Work out the finished part from the listing and answer in its coordinate system (mm). A direction names the side the tool comes from. Coordinates: 2 decimals unless noted, no trailing zeros. Order: outer loops, then holes, each group sorted by start corner. A loop starts at its lowest first (then second) coordinate and runs counter-clockwise, first axis right, second up. Notation, with made-up numbers: M -21,47 L -10,47 A26 cw -10,81 Z; hole C -0.75,48.25 d8. An arc over 180 degrees is marked long. Use a Markdown table: item, result.
Autodesk Inventor part; units mm, degrees
ref_plane "YZ Plane" through (0, 0, 0) normal (1, 0, 0) x (0, 1, 0)
ref_plane "XZ Plane" through (0, 0, 0) normal (0, 1, 0) x (-1, 0, 0)
ref_plane "XY Plane" through (0, 0, 0) normal (0, 0, 1) x (1, 0, 0)
sketch "スケッチ1" plane through (0, 0, 0) normal (0, 0, 1) x (1, 0, 0)
  line L0 (0, 0) -> (-28.77, 0)
  line L1 (-28.77, 0) -> (-28.77, -33.8125)
  line L2 (-28.77, -33.8125) -> (0, -33.8125)
  line L3 (0, -33.8125) -> (0, 0)
  circle A0 centre (-14.385, -28.04) radius 15.5
  line L4 (0, -4) -> (-5, 0)
  line L5 (-23.77, 0) -> (-28.77, -4)
  dimension "d0" = 28.77
  dimension "d2" = 31
  dimension "d4" = 4
  dimension "d5" = 4
  dimension "d6" = 5
  dimension "d7" = 5
  dimension "d66" = 28.04
extrude "押し出し1" add sketch "スケッチ1" along normal blind 9 contours L4 L3 A0 L1 L5 L0 | L3 L2 L1 A0 | A0 L2
sketch "スケッチ2" plane through (0, 0, 9) normal (0, 0, 1) x (1, 0, 0)
  line L0 (-5, 0) -> (-23.77, 0)
  arc A0 (-28.77, -33.8125) -> (0, -33.8125) centre (-14.385, -28.04) ccw
  point P0 (0, 0)
hole "穴1" at (-14.385, -28.04, 9) direction (0, 0, -1) diameter 8 end through all
sketch "スケッチ3" plane through (0, 0, 9) normal (0, 0, 1) x (1, 0, 0)
  line L0 (-28.77, -33.8125) -> (-38.2682, -31.1712)
  line L1 (-28.77, -22.086) -> (-38.3232, -24.9246)
  circle A0 centre (-37.3975, -28.04) radius 3.25
  circle A1 centre (-14.385, -28.04) radius 4
  line L2 (0, -33.8125) -> (9.4982, -31.1712)
  line L3 (0, -22.086) -> (9.5532, -24.9246)
  circle A2 centre (8.6275, -28.04) radius 3.25
  line L4 (-28.77, -4) -> (-28.77, -33.8125)
  line L5 (0, -33.8125) -> (0, -4)
  point P0 (0, 0)
  dimension "d19" = 5.954
  dimension "d20" = 6.5
  dimension "d53" = 46.025
  dimension "d54" = 23.0125
  dimension "d55" = 6.5
extrude "押し出し2" add sketch "スケッチ3" against normal blind 2.5 contours L0 A0 L1 L4 | A0 | L5 L3 A2 L2 | A2
sketch "スケッチ4" plane through (0, 0, 6.5) normal (0, 0, -1) x (-1, 0, 0)
  arc A0 (0, -33.8125) -> (28.77, -33.8125) centre (14.385, -28.04) ccw
  point P0 (0, 0)
  point P1 (30.6, -28.04)
  point P2 (-1.83, -28.04)
  dimension "d26" = 16.215
  dimension "d27" = 16.215
hole "穴2" at (-30.6, -28.04, 6.5) at (1.83, -28.04, 6.5) direction (0, 0, 1) diameter 3 end through all
sketch "スケッチ5" plane through (0, 0, 6.5) normal (0, 0, -1) x (-1, 0, 0)
  circle A0 centre (30.6, -28.04) radius 1.5
  circle A1 centre (-1.83, -28.04) radius 1.5
  point P0 (0, 0)
hole "穴3" at (-30.6, -28.04, 6.5) at (1.83, -28.04, 6.5) direction (0, 0, 1) diameter 5.6 depth 1.8
sketch "スケッチ6" plane through (0, 0, 6.5) normal (0, 0, -1) x (-1, 0, 0)
  circle A0 centre (14.385, -28.04) radius 4
  point P0 (0, 0)
  point P1 (37.3975, -28.04)
  point P2 (-8.6275, -28.04)
  dimension "d43" = 23.0125
  dimension "d45" = 23.0125
hole "穴4" at (-37.3975, -28.04, 6.5) at (8.6275, -28.04, 6.5) at (-14.385, -28.04, 6.5) direction (0, 0, 1) diameter 2.87 end through all
fillet "フィレット1" radius 0.4 4 edges at (-28.77, -4, 4.5) (-23.77, 0, 4.5) (-5, 0, 4.5) (0, -4, 4.5)
fillet "フィレット2" radius 0.5 10 edges at (-28.7305, -4.019, 0) (-26.2497, -1.9838, 0) (-23.7621, -0.0225, 0) (-14.385, 0, 0) (-5.0079, -0.0225, 0) (-2.5203, -1.9838, 0) (-0.0395, -4.019, 0) (0, -19.0024, 0) (-28.77, -19.0024, 0) (-14.385, -43.54, 0)
sketch "スケッチ7" plane through (-23.6297, 0, 9) normal (0, 1, 0) x (1, 0, 0)
  line L0 (3.2447, 5) -> (15.2447, 5)
  line L1 (15.2447, 5) -> (15.2447, 2)
  line L2 (15.2447, 2) -> (3.2447, 2)
  line L3 (3.2447, 2) -> (3.2447, 5)
  line L4 (18.4894, 0) -> (0, 0)
  point P0 (23.6297, 9)
  dimension "d60" = 3
  dimension "d61" = 12
  dimension "d62" = 8.385
  dimension "d63" = 2
extrude "押し出し3" add sketch "スケッチ7" along normal blind 5
equation "\"d4\" = d5"
equation "\"d6\" = d7"
equation "\"d54\" = 0.5 * d53"
equation "\"d55\" = d20"
properties part number "AMT102-V"
1. Find the intervals of material crossed by probe 1 along X at (y, z) = (-28.04, 8.6) (1 decimal); probe 2 along X at (y, z) = (-28.04, 7.05) (1 decimal); probe 3 along Y at (x, z) = (-30.6, 7.9), in increasing order.
Answers below:
| item | result |
|---|---|
| probe 1 | -40.6 to -38.8, -36 to -32.1, -29.1 to -18.4, -10.4 to 0.3, 3.3 to 7.2, 10.1 to 11.9 |
| probe 2 | -40.6 to -38.8, -36 to -33.4, -27.8 to -18.4, -10.4 to -1, 4.6 to 7.2, 10.1 to 11.9 |
| probe 3 | -33.3 to -30.84, -25.24 to -22.63 |
2. For faces 5 (the face through (-14, 2, 4)), 6 (the face through (-8.385, 2, 5)), 7 (the face through (-20.385, 2, 6)), 8 (the face through (6, -28, 6.5)), determine the directions among +Z, -Z, +X, -X, +Y, -Y from which every point of the face is accessible in a straight line to the end or side of a thin tool.
Answers below:
| item | result |
|---|---|
| face 5 | -Z, +X, -X, +Y |
| face 6 | +Z, -Z, +X, +Y |
| face 7 | +Z, -Z, -X, +Y |
| face 8 | -Z, +X, +Y, -Y |
3. Section A-A on y = -28.04 is taken. Give the number of separate pieces and of enclosed holes in the cut face, then the cut area to 4 significant figures.
Answers below:
| item | result |
|---|---|
| separate pieces | 6 |
| enclosed holes | 0 |
| area | 207.5 mm² |
4. Section C-C on x = 1.83 is taken. Determine the outline of the cut face in (y, z).
Answers below:
| item | result |
|---|---|
| outline | M -33.3,6.5 L -30.84,6.5 L -30.84,8.3 L -29.54,8.3 L -29.54,9 L -33.3,9 Z; M -26.54,8.3 L -25.24,8.3 L -25.24,6.5 L -22.63,6.5 L -22.63,9 L -26.54,9 Z |
5. Section D-D on y = 2.5 is taken. Determine the outline of the cut face in (x, z) (3 decimals), then the cut area to 3 significant figures.
Answers below:
| item | result |
|---|---|
| outline | M -20.385,4 L -8.385,4 L -8.385,7 L -20.385,7 Z |
| area | 36.0 mm² |
6. Flat-ended cylindrical pins translate along their axes: P1, Ø1.7, axis at x = 3, y = -27, coming from the -Z side; P2, Ø2.5, axis at x = -14.5, y = 3, coming from the +Z side; P3, Ø3.5, axis at y = 3.5, z = 5, coming from the +X side (3 decimals). Find the tip coordinate at first contact, or state that the pin passes through.
Answers below:
| item | result |
|---|---|
| P1 | z = 8.3 |
| P2 | z = 7 |
| P3 | x = -8.385 |
7. For a pull along X with two mould halves and no side action, classify faces 1 (the face through (4.68, -32.51, 7.77)), 2 (the face through (-35, -28, 6.5)), 3 (the face through (-30.67, -29.54, 8.65)), 4 (the face through (-28, -27, 7)) as +X half, -X half, draft (parallel to the pull), parting line (faces both ways), or undercut.
Answers below:
| item | result |
|---|---|
| face 1 | +X half |
| face 2 | draft |
| face 3 | undercut |
| face 4 | undercut |
